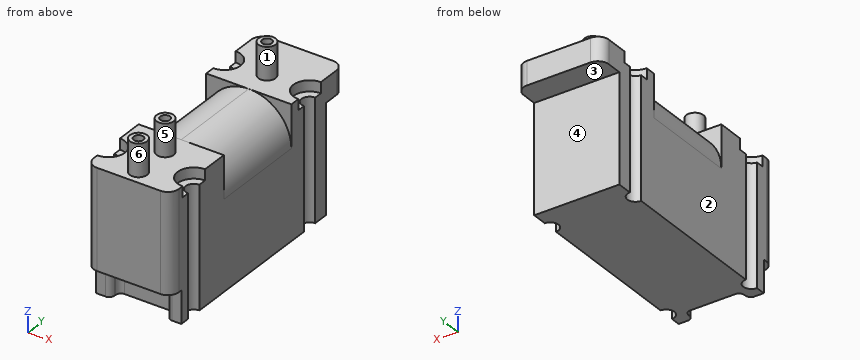
```python
from build123d import *

# Parameters (mm, degrees)
SKETCH1_W           = 7.87
SKETCH1_H           = 23
BOSS_EXTRUDE1_DEPTH = 12.19
SKETCH2_R           = 0.79375
BOSS_EXTRUDE2_DEPTH = 3
SKETCH3_R           = 0.75
CUT_EXTRUDE1_DEPTH  = 12.19
FILLET1_R           = 1
SKETCH4_R           = 1.5
CUT_EXTRUDE2_DEPTH  = 1
SKETCH5_W           = 7.87
SKETCH5_H           = 2.41
CUT_EXTRUDE3_DEPTH  = 10
CUT_EXTRUDE4_START  = -3
CUT_EXTRUDE4_DEPTH  = 3
SKETCH7_R           = 0.45
CUT_EXTRUDE5_DEPTH  = 8
CUT_EXTRUDE6_DEPTH  = 9


with BuildPart() as part:
    # Sketch1 → Boss-Extrude1 (new body)
    with BuildSketch(Plane.XY):
        with Locations((3.935, 11.5)):
            Rectangle(SKETCH1_W, SKETCH1_H)
    extrude(amount=BOSS_EXTRUDE1_DEPTH)

    # Sketch2 → Boss-Extrude2 (add)
    with BuildSketch(Plane.XY.offset(12.19)):
        with Locations(Location((3.935, 18.43, 0), (0, 0, 180))):
            Circle(SKETCH2_R)
        with Locations(Location((3.935, 4.854367324, 0), (0, 0, 180))):
            Circle(SKETCH2_R)
        with Locations(Location((3.935, 1.31, 0), (0, 0, 180))):
            Circle(SKETCH2_R)
    extrude(amount=BOSS_EXTRUDE2_DEPTH)

    # Sketch3 → Cut-Extrude1 (cut)
    with BuildSketch(Plane.XY.offset(12.19)):
        with Locations((0, 18.43)):
            Circle(SKETCH3_R)
        with Locations((0, 3)):
            Circle(SKETCH3_R)
        with Locations((7.87, 3)):
            Circle(SKETCH3_R)
        with Locations((7.87, 18.43)):
            Circle(SKETCH3_R)
    extrude(amount=-CUT_EXTRUDE1_DEPTH, mode=Mode.SUBTRACT)

    # Fillet1
    fillet1_edges = [part.edges().sort_by_distance(p)[0] for p in [
        (0, 23, 6.095),
        (7.87, 23, 6.095),
        (7.87, 0, 6.095),
        (0, 0, 6.095),
    ]]
    fillet(fillet1_edges, radius=FILLET1_R)

    # Sketch4 → Cut-Extrude2 (cut)
    with BuildSketch(Plane.XY.offset(12.19)):
        with Locations((0, 18.43)):
            Circle(SKETCH4_R)
        with Locations((0, 3)):
            Circle(SKETCH4_R)
        with Locations((7.87, 3)):
            Circle(SKETCH4_R)
        with Locations((7.87, 18.43)):
            Circle(SKETCH4_R)
    extrude(amount=-CUT_EXTRUDE2_DEPTH, mode=Mode.SUBTRACT)

    # Sketch5 → Cut-Extrude3 (cut)
    with BuildSketch(Plane(origin=(0, 0, 0), x_dir=(-1, 0, 0), z_dir=(0, 0, -1))):
        with Locations((-3.935, 21.795)):
            Rectangle(SKETCH5_W, SKETCH5_H)
    extrude(amount=-CUT_EXTRUDE3_DEPTH, mode=Mode.SUBTRACT)

    # Sketch6 → Cut-Extrude4 (cut)
    with BuildSketch(Plane(origin=(0, 0, 0), x_dir=(-1, 0, 0), z_dir=(0, 0, -1)).offset(CUT_EXTRUDE4_START)):
        with BuildLine():
            Line((-7.87, 1.349131469), (-7.01383854, 1.349131469))
            ThreePointArc((-7.01383854, 1.349131469), (-6.660285149, 1.495578078), (-6.51383854, 1.849131469))
            Line((-6.51383854, 1.849131469), (-6.51383854, 1.968890308))
            ThreePointArc((-6.51383854, 1.968890308), (-6.36739193, 2.322443699), (-6.01383854, 2.468890308))
            Line((-6.01383854, 2.468890308), (-1.85616146, 2.468890308))
            ThreePointArc((-1.85616146, 2.468890308), (-1.50260807, 2.322443699), (-1.35616146, 1.968890308))
            Line((-1.35616146, 1.968890308), (-1.35616146, 1.849131469))
            ThreePointArc((-1.35616146, 1.849131469), (-1.209714851, 1.495578078), (-0.85616146, 1.349131469))
            Line((-0.85616146, 1.349131469), (0, 1.349131469))
            Line((0, 1.349131469), (0, 1))
            ThreePointArc((0, 1), (-0.292893219, 0.292893219), (-1, 0))
            Line((-1, 0), (-6.87, 0))
            ThreePointArc((-6.87, 0), (-7.577106781, 0.292893219), (-7.87, 1))
            Line((-7.87, 1), (-7.87, 1.349131469))
        make_face()
    extrude(amount=CUT_EXTRUDE4_DEPTH, mode=Mode.SUBTRACT)

    # Sketch7 → Cut-Extrude5 (cut)
    with BuildSketch(Plane.XY.offset(15.19)):
        with Locations((3.935, 18.43)):
            Circle(SKETCH7_R)
        with Locations((3.935, 4.854367324)):
            Circle(SKETCH7_R)
        with Locations((3.935, 1.31)):
            Circle(SKETCH7_R)
    extrude(amount=-CUT_EXTRUDE5_DEPTH, mode=Mode.SUBTRACT)

    # Sketch8 → Cut-Extrude6 (cut)
    with BuildSketch(Plane(origin=(0, 7, 0), x_dir=(-1, 0, 0), z_dir=(0, -1, 0))):
        with BuildLine():
            Line((0, -12.19), (0, -8.255))
            ThreePointArc((0, -8.255), (-1.152534816, -11.037465184), (-3.935, -12.19))
            Line((-3.935, -12.19), (0, -12.19))
        make_face()
        with BuildLine():
            Line((-7.87, -12.19), (-3.935, -12.19))
            ThreePointArc((-3.935, -12.19), (-6.717465184, -11.037465184), (-7.87, -8.255))
            Line((-7.87, -8.255), (-7.87, -12.19))
        make_face()
    extrude(amount=-CUT_EXTRUDE6_DEPTH, mode=Mode.SUBTRACT)


solid = part.part
```
Here's how the part is built. I have some questions about the finished solid (model axes, mm). Face numbers are marked on the shaded views. A direction names the side the tool comes from. Round coordinates to 2 decimals unless told otherwise and drop trailing zeros. Order: outer loops, then holes, each group sorted by start corner. A loop starts at its lowest first (then second) coordinate and runs counter-clockwise, first axis right, second up. Notation, with made-up numbers: (55, 26) -> (75, 26) arc R17 ccw to (75, 46) -> close; hole circle Ø1 at (56, 72). An arc over 180 degrees is marked (long way). Use a Markdown table: item, result. Add a question column.
(1) For pin 1 Ø1.2 at (x, y) = (3, 0.5) entering from -Z; pin 2 Ø0.5 at (x, y) = (1, 19) entering from +Z; pin 3 Ø0.7 at (x, y) = (3.5, 21.5) entering from -Z, each with a flat end and sliding along its axis, tell me the tip position at first contact or that it passes through.
(2) Suppose I cut it at C-C, the plane x = 5. Please give me the cut outline in (y, z).
(3) Suppose I cut it at D-D, the plane y = 3. Please give me the cut outline in (x, z).
(4) I need wall thicknesses on line 1 along Y through (x, z) = (4, 11.25); line 2 along X through (y, z) = (18.43, 13) (3 decimals); line 3 along Y through (x, z) = (7.75, 5.5). Which ranges of each line are inside material? Lowest first, please.
(5) If we mould it in two halves opening along Y, with no side actions, what happens to the marked faces 3, 4, 5 and 6? For each: released by +Y, released by -Y, zero draft, split by the parting line, or undercut.
(6) Suppose I cut it at A-A, the plane z = 8. Please give me the cut outline in (x, y) (3 decimals), and give its area (3 significant figures).
(7) For the marked faces 1 and 2, which set-ups out of +Z, -Z, +X, -X, +Y, -Y let a thin tool reach every point of the face, with its end or its side?
(8) Suppose I cut it at B-B, the plane y = 7.5. Please give me the cut outline in (x, z) (3 decimals), and give its area (3 significant figures).
Verdict:
| question | item | result |
|---|---|---|
| 1 | pin 1 | z = 3 |
| 1 | pin 2 | z = 11.19 |
| 1 | pin 3 | z = 10 |
| 2 | outline | (0, 3) -> (2.47, 3) -> (2.47, 0) -> (20.59, 0) -> (20.59, 10) -> (23, 10) -> (23, 12.19) -> (16, 12.19) -> (16, 12.04) -> (7, 12.04) -> (7, 12.19) -> (0, 12.19) -> close |
| 3 | outline | (0.75, 0) -> (7.12, 0) -> (7.12, 11.19) -> (6.37, 11.19) -> (6.37, 12.19) -> (1.5, 12.19) -> (1.5, 11.19) -> (0.75, 11.19) -> close |
| 4 | line 1 | 0 to 0.86, 1.76 to 4.41, 5.3 to 17.98, 18.88 to 23 |
| 4 | line 2 | 3.141 to 3.485, 4.385 to 4.729 |
| 4 | line 3 | 0.53 to 2.26, 3.74 to 17.69, 19.17 to 20.59 |
| 5 | face 3 | zero draft |
| 5 | face 4 | released by +Y |
| 5 | face 5 | undercut |
| 5 | face 6 | undercut |
| 6 | outline | (0, 1) arc R1 ccw to (1, 0) -> (6.87, 0) arc R1 ccw to (7.87, 1) -> (7.87, 2.25) arc R0.75 cw to (7.87, 3.75) -> (7.87, 17.68) arc R0.75 cw to (7.87, 19.18) -> (7.87, 20.59) -> (0, 20.59) -> (0, 19.18) arc R0.75 cw to (0, 17.68) -> (0, 3.75) arc R0.75 cw to (0, 2.25) -> close; hole circle Ø0.9 at (3.935, 1.31); hole circle Ø0.9 at (3.935, 4.854); hole circle Ø0.9 at (3.935, 18.43) |
| 6 | area | 156 mm2 |
| 7 | face 1 | +Z |
| 7 | face 2 | +Z, -Z, -X, +Y, -Y |
| 8 | outline | (0, 0) -> (7.87, 0) -> (7.87, 8.255) arc R3.935 ccw to (0, 8.255) -> close |
| 8 | area | 89.3 mm2 |
